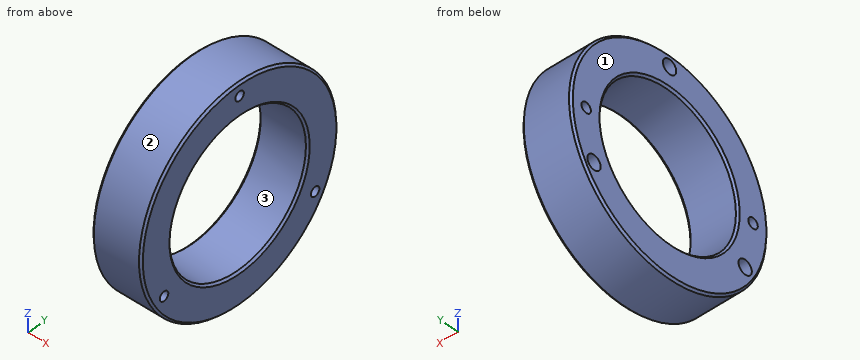
from build123d import *

# Parameters (mm, degrees)
SKETCH1_W           = 25.3746
SKETCH1_H           = 38.1
CHAMFER1_SIZE       = 1.524
SKETCH2_R           = 3.5687
CUT_EXTRUDE2_DEPTH  = 76.2
SKETCH3_R           = 5.5626
CUT_EXTRUDE4_DEPTH  = 9.652
SKETCH4_R           = 3.5687
CUT_EXTRUDE6_DEPTH  = 76.2
SKETCH5_R           = 5.5626
CUT_EXTRUDE8_DEPTH  = 9.652
SKETCH6_R           = 3.5687
CUT_EXTRUDE10_DEPTH = 76.2
SKETCH7_R           = 5.5626
CUT_EXTRUDE12_DEPTH = 9.652
SKETCH8_R           = 3.96875
CUT_EXTRUDE14_DEPTH = 25.4
SKETCH9_R           = 3.96875
CUT_EXTRUDE16_DEPTH = 25.4


with BuildPart() as part:
    # Sketch1 → Revolve1 (revolve)
    with BuildSketch(Plane(origin=(0, 0, 0), x_dir=(0, 1, 0), z_dir=(0, 0, 1)), mode=Mode.PRIVATE) as revolve1_sk:
        with Locations((69.8373, -19.05)):
            Rectangle(SKETCH1_W, SKETCH1_H)
    revolve(revolve1_sk.sketch.rotate(Axis((-25.4, 0, 0), (1, 0, 0)), 90), axis=Axis((-25.4, 0, 0), (1, 0, 0)))

    # Chamfer1
    chamfer1_edges = [part.edges().sort_by_distance(p)[0] for p in [
        (0, 0, -57.15),
        (38.1, 0, -57.15),
        (38.1, 0, -82.5246),
        (0, 0, -82.5246),
    ]]
    chamfer(chamfer1_edges, length=CHAMFER1_SIZE)

    # Sketch2 → Cut-Extrude2 (cut)
    with BuildSketch(Plane.YZ):
        with Locations(Location((0, 73.025, 0), (0, 0, 90))):
            Circle(SKETCH2_R)
    extrude(amount=CUT_EXTRUDE2_DEPTH, mode=Mode.SUBTRACT)

    # Sketch3 → Cut-Extrude4 (cut)
    with BuildSketch(Plane.YZ):
        with Locations(Location((0, 73.025, 0), (0, 0, 270))):
            Circle(SKETCH3_R)
    extrude(amount=CUT_EXTRUDE4_DEPTH, mode=Mode.SUBTRACT)

    # Sketch4 → Cut-Extrude6 (cut)
    with BuildSketch(Plane.YZ):
        with Locations(Location((-63.246, -36.5252, 0), (0, 0, 90))):
            Circle(SKETCH4_R)
    extrude(amount=CUT_EXTRUDE6_DEPTH, mode=Mode.SUBTRACT)

    # Sketch5 → Cut-Extrude8 (cut)
    with BuildSketch(Plane.YZ):
        with Locations(Location((-63.246, -36.5252, 0), (0, 0, 270))):
            Circle(SKETCH5_R)
    extrude(amount=CUT_EXTRUDE8_DEPTH, mode=Mode.SUBTRACT)

    # Sketch6 → Cut-Extrude10 (cut)
    with BuildSketch(Plane.YZ):
        with Locations(Location((63.246, -36.5252, 0), (0, 0, 90))):
            Circle(SKETCH6_R)
    extrude(amount=CUT_EXTRUDE10_DEPTH, mode=Mode.SUBTRACT)

    # Sketch7 → Cut-Extrude12 (cut)
    with BuildSketch(Plane.YZ):
        with Locations(Location((63.246, -36.5252, 0), (0, 0, 270))):
            Circle(SKETCH7_R)
    extrude(amount=CUT_EXTRUDE12_DEPTH, mode=Mode.SUBTRACT)

    # Sketch8 → Cut-Extrude14 (cut)
    with BuildSketch(Plane.YZ):
        with Locations(Location((-69.85, 0, 0), (0, 0, 270))):
            Circle(SKETCH8_R)
    extrude(amount=CUT_EXTRUDE14_DEPTH, mode=Mode.SUBTRACT)

    # Sketch9 → Cut-Extrude16 (cut)
    with BuildSketch(Plane.YZ):
        with Locations(Location((69.85, 0, 0), (0, 0, 270))):
            Circle(SKETCH9_R)
    extrude(amount=CUT_EXTRUDE16_DEPTH, mode=Mode.SUBTRACT)


solid = part.part
Input: part model. Units: mm. Frame: model coordinates. Face numbers are marked on the shaded views. Coordinates: 2 decimals unless noted, no trailing zeros. Loops run counter-clockwise (first coordinate to the right, second up) from the corner with the lowest first, then second, coordinate; pieces in that order, holes last. Notation, with made-up numbers: (70.5, 54.5) - (122.5, 54.5) arc R22 ccw to (122.5, 69.5) - close; hole circle Ø2 at (59.25, 38). An arc over 180 degrees is marked (long way). Answer in a Markdown table with one row per item. Add a question column.
Item 1: Contact query for flat-ended pins moving along their axis: P1, Ø1.5, axis at x = 6, z = -17.5, coming from the -Y side; P2, Ø9.5, axis at y = 63.25, z = -36.53, coming from the -X side; P3, Ø6, axis at x = 32.5, y = -25, coming from the +Z side; P4, Ø4.5, axis at y = -63.25, z = -36.53, coming from the -X side. Output: stop coordinate, or through.
Item 2: Mould query, pull axis Z, two halves, no side actions, for the marked faces 1, 2 and 3. Classes: released by +Z, released by -Z, zero draft, split by the parting line, or undercut.
Item 3: Section query A-A on y = 0. Return the cut outline in (x, z).
Item 4: Line query: line 1 along Y through (x, z) = (10, 0); line 2 along Z through (x, y) = (29.5, 11.5); line 3 along Y through (x, z) = (25, 20). Output: solid intervals per line, ascending. Write a range as [from, to].
Item 5: Section query B-B on z = 0. Return the cut outline in (x, y), then the cut area to 3 significant figures.
Item 6: Section query C-C on x = 4.5. State how many separate pieces and enclosed holes the cut face has, then the cut area to 3 significant figures.
Recorded:
| question | item | result |
|---|---|---|
| 1 | P1 | y = -80.81 |
| 1 | P2 | x = 9.65 |
| 1 | P3 | z = 79.54 |
| 1 | P4 | through |
| 2 | face 1 | zero draft |
| 2 | face 2 | split by the parting line |
| 2 | face 3 | undercut |
| 3 | outline | (0, -81) - (1.52, -82.52) - (36.58, -82.52) - (38.1, -81) - (38.1, -58.67) - (36.58, -57.15) - (1.52, -57.15) - (0, -58.67) - close; (0, 58.67) - (1.52, 57.15) - (36.58, 57.15) - (38.1, 58.67) - (38.1, 69.46) - (9.65, 69.46) - (9.65, 67.46) - (0, 67.46) - close; (0, 78.59) - (9.65, 78.59) - (9.65, 76.59) - (38.1, 76.59) - (38.1, 81) - (36.58, 82.52) - (1.52, 82.52) - (0, 81) - close |
| 4 | line 1 | [-82.52, -73.82], [-65.88, -57.15], [57.15, 65.88], [73.82, 82.52] |
| 4 | line 2 | [-81.72, -55.98], [55.98, 81.72] |
| 4 | line 3 | [-80.06, -53.54], [53.54, 80.06] |
| 5 | outline | (0, -81) - (1.52, -82.52) - (36.58, -82.52) - (38.1, -81) - (38.1, -58.67) - (36.58, -57.15) - (1.52, -57.15) - (0, -58.67) - (0, -65.88) - (25.4, -65.88) - (25.4, -73.82) - (0, -73.82) - close; (0, 58.67) - (1.52, 57.15) - (36.58, 57.15) - (38.1, 58.67) - (38.1, 81) - (36.58, 82.52) - (1.52, 82.52) - (0, 81) - (0, 73.82) - (25.4, 73.82) - (25.4, 65.88) - (0, 65.88) - close |
| 5 | area | 1,520 mm^2 |
| 6 | separate pieces | 1 |
| 6 | enclosed holes | 6 |
| 6 | area | 10,700 mm^2 |
